The model under review builds one solid part; all positions refer to its coordinate system, in mm. A direction names the side the tool comes from. Coordinates: 2 decimals unless noted, no trailing zeros. Order: outer loops, then holes, each group sorted by start corner. A loop starts at its lowest first (then second) coordinate and runs counter-clockwise, first axis right, second up. Notation, with made-up numbers: (64.25, 62) -> (100.25, 62) arc R33 ccw to (100.25, 98) -> close; hole circle Ø6 at (55, 87.5). An arc over 180 degrees is marked (long way). Use one line per item in the form item = value.
from build123d import *

# Parameters (mm, degrees)
PAD_DEPTH       = 40
SKETCH001_W     = 37
SKETCH001_H     = 36
POCKET_DEPTH    = 38
SKETCH002_R     = 6.5
POCKET001_DEPTH = 5
SKETCH003_R     = 2
POCKET002_DEPTH = 5
CHAMFER_SIZE    = 1


with BuildPart() as part:
    # Sketch → Pad (new body)
    with BuildSketch(Plane.XZ):
        Polygon((0, 0), (-40, 0), (-40, 40), align=None)
    extrude(amount=PAD_DEPTH)

    # Sketch001 (on DatumPlane) → Pocket (cut)
    with BuildSketch(Plane.XY.offset(40)):
        with Locations((-18.5, -20.771839)):
            Rectangle(SKETCH001_W, SKETCH001_H)
    extrude(amount=-POCKET_DEPTH, mode=Mode.SUBTRACT)

    # Sketch002 (on Face3 of Pocket) → Pocket001 (cut)
    with BuildSketch(Plane(origin=(-40, 0, 0), x_dir=(0, 0, -1), z_dir=(-1, 0, 0))):
        with Locations((-20, 20)):
            Circle(SKETCH002_R)
    extrude(amount=-POCKET001_DEPTH, mode=Mode.SUBTRACT)

    # Sketch003 (on Face9 of Pocket001) → Pocket002 (cut)
    with BuildSketch(Plane(origin=(0, 0, 2), x_dir=(-1, 0, 0), z_dir=(0, 0, 1))):
        with Locations((32, 33.771839)):
            Circle(SKETCH003_R)
        with Locations((7, 7.771839)):
            Circle(SKETCH003_R)
        with Locations((7, 33.771839)):
            Circle(SKETCH003_R)
        with Locations((32, 7.771839)):
            Circle(SKETCH003_R)
    extrude(amount=-POCKET002_DEPTH, mode=Mode.SUBTRACT)

    # Chamfer
    chamfer_edges = [part.edges().sort_by_distance(p)[0] for p in [
        (-30, -33.771839, 2),
        (-30, -7.771839, 2),
        (-5, -7.771839, 2),
        (-5, -33.771839, 2),
    ]]
    chamfer(chamfer_edges, length=CHAMFER_SIZE)


solid = part.part
Item 1: Draft analysis for pull direction Y (two halves, no side actions). For faces 1 (the face through (-28, -2.772, 12)), 2 (the face through (-20, -20, 0)), 3 (the face through (-29, -40, 11)), state which applies: released by +Y, released by -Y, zero draft, split by the parting line, or undercut.
Results found:
face_1 = undercut
face_2 = zero draft
face_3 = released by -Y
Item 2: We need section B-B (y = -17.5). Write out the cut boundary in (x, z).
Results found:
outline = (-40, 0) -> (0, 0) -> (-2, 2) -> (-37, 2) -> (-37, 14) -> (-40, 14) -> close; (-40, 26) -> (-37, 26) -> (-37, 37) -> (-40, 40) -> close
Item 3: We need section A-A (x = -7). Write out the cut boundary in (y, z), plus the area to 3 significant figures.
Results found:
outline = (-40, 0) -> (-35.77, 0) -> (-35.77, 1) -> (-36.77, 2) -> (-38.77, 2) -> (-38.77, 7) -> (-40, 7) -> close; (-31.77, 0) -> (-9.77, 0) -> (-9.77, 1) -> (-10.77, 2) -> (-30.77, 2) -> (-31.77, 1) -> close; (-5.77, 0) -> (0, 0) -> (0, 7) -> (-2.77, 7) -> (-2.77, 2) -> (-4.77, 2) -> (-5.77, 1) -> close
area = 82.0 mm²
Item 4: We need section D-D (z = 34). Write out the cut boundary in (x, y), plus the area to 3 significant figures.
Results found:
outline = (-40, -40) -> (-34, -40) -> (-34, -38.77) -> (-37, -38.77) -> (-37, -2.77) -> (-34, -2.77) -> (-34, 0) -> (-40, 0) -> close
area = 132 mm²
Item 5: To check wall thickness, follow L1, parallel to Y at x = -38, z = 20; L2, parallel to Y at x = -22.5, z = 6.5; L3, parallel to X at y = -28, z = 24. State the ranges of each line that lie inside material, in increasing order. Write a range as from..to.
Results found:
L1 = -40..-26.5, -13.5..0
L2 = -40..-38.77, -2.77..0
L3 = -40..-37
Item 6: Clearance check with flat-ended pins moving along their axes: pin 1 (5 mm diameter, centred on x = -7, y = -33.77, fed in from +Z); pin 2 (10.5 mm diameter, centred on y = -13.5, z = 22, fed in from +X); pin 3 (3.5 mm diameter, centred on x = -32, y = -7.77, fed in from -Z). State where each tip first meets the part, or that it passes through.
Results found:
pin_1 = 1.5
pin_2 = -37
pin_3 = through
Item 7: Tool access review of faces 4 (the face through (-20, -21, 2)), 5 (the face through (-5.526, -9.124, 0.507)): name each direction out of +Z, -Z, +X, -X, +Y, -Y from which nothing blocks a thin tool from reaching the whole face with its end or side.
Results found:
face_4 = +Z, +X
face_5 = +Z, -Z
Item 8: We need section C-C (z = 20). Write out the cut boundary in (x, y), plus the area to 3 significant figures.
Results found:
outline = (-40, -40) -> (-20, -40) -> (-20, -38.77) -> (-37, -38.77) -> (-37, -26.5) -> (-40, -26.5) -> close; (-40, -13.5) -> (-37, -13.5) -> (-37, -2.77) -> (-20, -2.77) -> (-20, 0) -> (-40, 0) -> close
area = 149 mm²
